Geometry check sheet. Reference: drawing and pictorial views, mm from the part's lowest x, y, z. Round coordinates to 2 decimals unless told otherwise and drop trailing zeros. Write each loop counter-clockwise with the first axis right and the second up, starting at its lowest first coordinate (ties: lowest second). Pieces come first, ordered by that corner, then holes. Notation, with made-up numbers: (13.25, -14.75) - (49.25, -14.75) arc R27 ccw to (49.25, 14.25) - close; hole circle Ø3 at (59.25, -35.5). An arc over 180 degrees is marked (long way). Use one line per item in the form item = value. Start each with the question number.
1) Section check C-C (z = 27). Record the boundary of the cut face in (x, y) (1 decimal).
2) Scan lines: probe 1 along Z at (x, y) = (0.6, 2); probe 2 along Y at (x, z) = (2.85, 27.5) (1 decimal); probe 3 along Y at (x, z) = (1.15, 28) (1 decimal). Record each from-to range of solid material in increasing order.
3) Section check D-D (y = 17). Count the separate pieces of the cut face and the enclosed holes in it.
4) Gauge pin test, flat ends, axial feed: P1, Ø1.6, axis at x = 1, y = 14.5, coming from the -Z side (1 decimal); P2, Ø1, axis at x = 1, z = 11.5, coming from the -Y side (1 decimal). Record the tip position at first contact, or that the pin passes through.
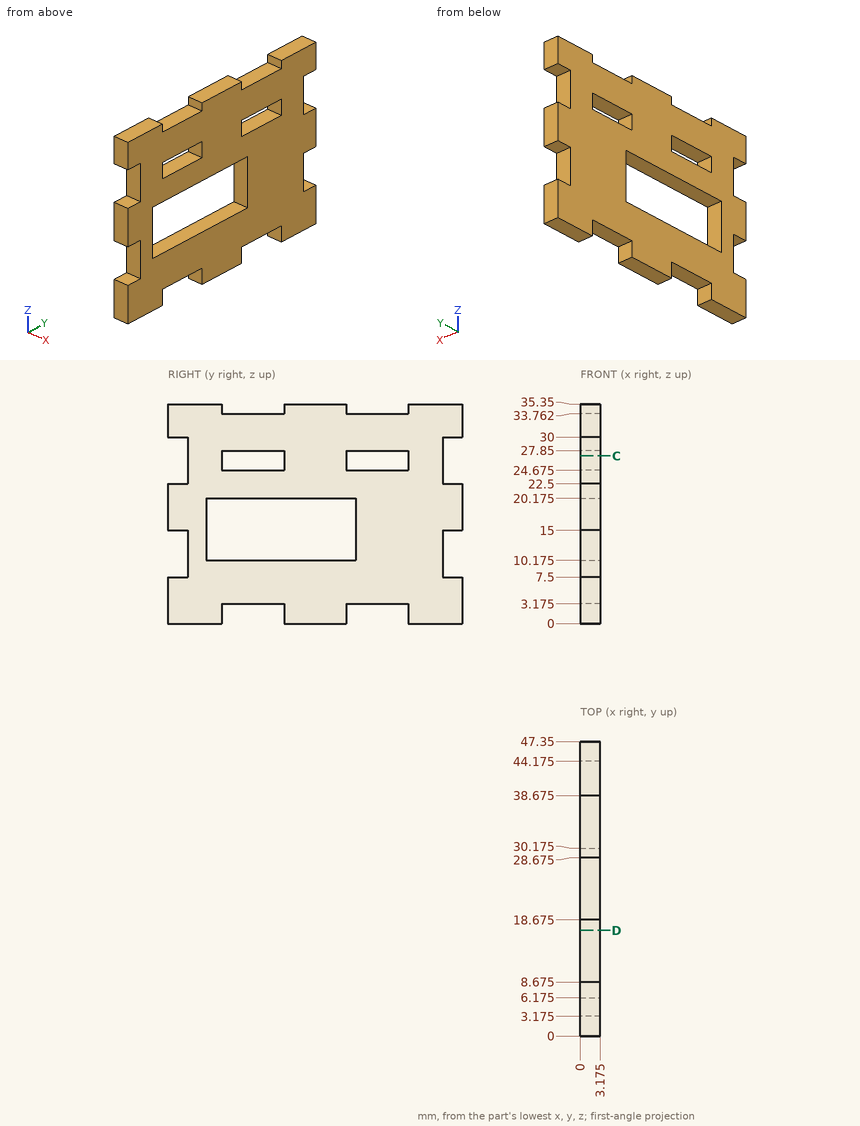
Results are:
q1.outline = (0, 3.2) - (3.2, 3.2) - (3.2, 8.7) - (0, 8.7) - close; (0, 18.7) - (3.2, 18.7) - (3.2, 28.7) - (0, 28.7) - close; (0, 38.7) - (3.2, 38.7) - (3.2, 44.2) - (0, 44.2) - close
q2.probe_1 = 0 to 7.5, 15 to 22.5, 30 to 35.35
q2.probe_2 = 3.2 to 8.7, 18.7 to 28.7, 38.7 to 44.2
q2.probe_3 = 3.2 to 44.2
q3.separate_pieces = 3
q3.enclosed_holes = 0
q4.P1 = 3.2
q4.P2 = 3.2
